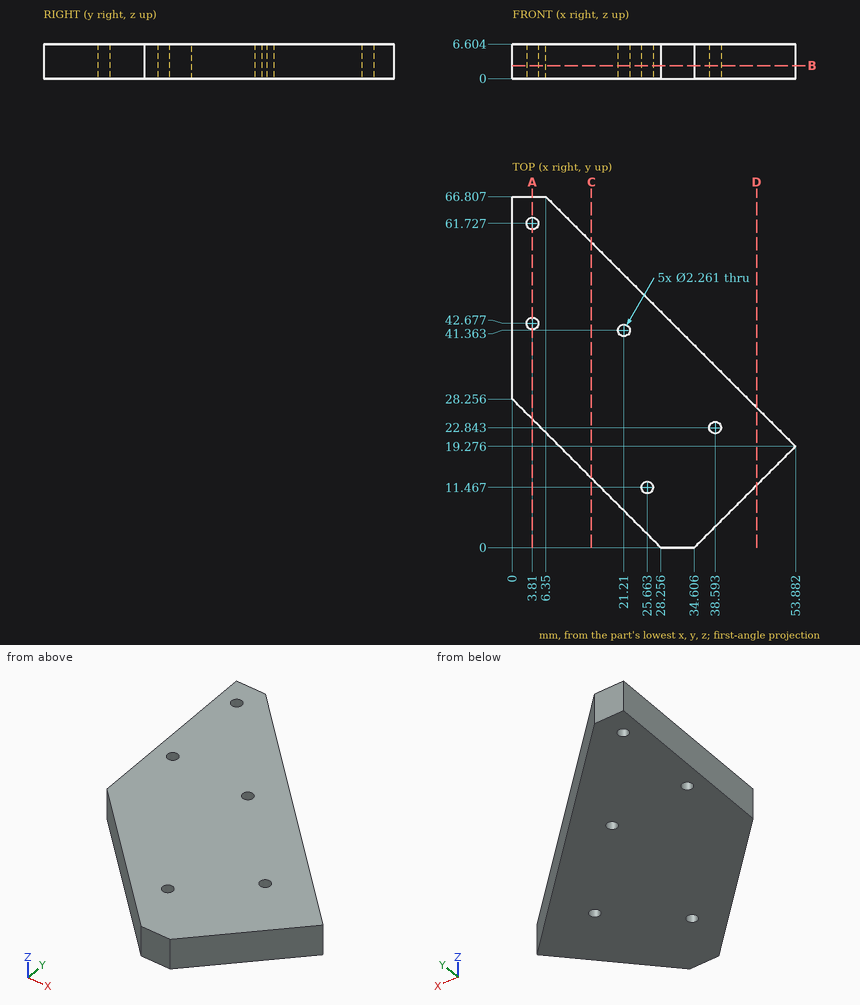
Study the drawing (mm; zero at the part's minimum x, y, z) and answer. Give positions to 0.01 mm unless a question says otherwise; leave off trailing zeros. Loops run counter-clockwise (first coordinate to the right, second up) from the corner with the lowest first, then second, coordinate; pieces in that order, holes last. Notation, with made-up numbers: (58.25, 27) - (89.25, 27) arc R19 cw to (89.25, 61) - close; hole circle Ø11 at (75, 67). An arc over 180 degrees is marked (long way). Return JSON: item names as keys, results as strings. Group by question number.
1. Find section B-B (z = 2.5). State how many separate pieces and enclosed holes the cut face has, then the cut area to 4 significant figures.
2. Find section A-A (x = 3.81). Write down the section's boundary in (y, z) (1 decimal).
3. Find section D-D (x = 46.5). Write down the section's boundary in (y, z) (1 decimal), then the cut area to 3 significant figures.
4. Given pin 1 Ø1 at (y, z) = (21.5, 5) entering from -X (1 decimal); pin 2 Ø3 at (x, y) = (21.21, 41.36) entering from +Z; pin 3 Ø1 at (x, z) = (41.5, 4.5) entering from +Y, each flat-ended and moving along its own axis, determine where each tip first touches the part or whether it passes through.
5. Find section C-C (x = 15). Write down the section's boundary in (y, z) (1 decimal).
6. Straight lines are drawn through the part: line 1 (Y direction, x = 4, z = 3.75) (1 decimal); line 2 (Y direction, x = 3.81, z = 1.5) (1 decimal); line 3 (X direction, y = 42, z = 3.5) (1 decimal). For each, find the intervals that lie inside material, in ascending order. Write a range as [from, to].
Verdict:
{
 "1": {"separate pieces": "1", "enclosed holes": "5", "area": "1,865 mm^2"},
 "2": {"outline": "(24.4, 0) - (41.5, 0) - (41.5, 6.6) - (24.4, 6.6) - close; (43.8, 0) - (60.6, 0) - (60.6, 6.6) - (43.8, 6.6) - close; (62.9, 0) - (66.8, 0) - (66.8, 6.6) - (62.9, 6.6) - close"},
 "3": {"outline": "(11.9, 0) - (26.7, 0) - (26.7, 6.6) - (11.9, 6.6) - close", "area": "97.5 mm^2"},
 "4": {"pin 1": "stops at x = 6.3", "pin 2": "stops at z = 6.6", "pin 3": "stops at y = 32.16"},
 "5": {"outline": "(13.3, 0) - (58.2, 0) - (58.2, 6.6) - (13.3, 6.6) - close"},
 "6": {"line 1": "y = [24.3, 41.6], [43.8, 60.6], [62.8, 66.8]", "line 2": "y = [24.4, 41.5], [43.8, 60.6], [62.9, 66.8]", "line 3": "x = [0, 2.9], [4.7, 20.3], [22.1, 31.2]"}
}
